Design review of the part built by this model. Coordinates are the model's own, in mm. Coordinates: 2 decimals unless noted, no trailing zeros. Loops run counter-clockwise (first coordinate to the right, second up) from the corner with the lowest first, then second, coordinate; pieces in that order, holes last. Notation, with made-up numbers: M -35.5,-24 L 10.5,-24 A36 cw 10.5,15 Z; hole C 59,86 d5. An arc over 180 degrees is marked long. Write item = value, one per line. Start each with the question number.
from build123d import *

# Parameters (mm, degrees)
F0_R     = 15.875
F0_R_2   = 11.25
F1_DEPTH = 38
F3_R     = 4
F4_DEPTH = 15.876


# Not quite as in the source:
# - a fillet or chamfer that OpenCascade refuses, or shapes differently, is made with other operations: its cross-section is extruded or revolved along the edge and cut away or added


with BuildPart() as f1:
    # F0 (on Top) → F1 (new body)
    with BuildSketch(Plane.XY):
        Circle(F0_R)
        Circle(F0_R_2, mode=Mode.SUBTRACT)
    extrude(amount=F1_DEPTH)

    # F2: fillet of radius 5 on 2 edges, made by hand

    # F2_s1 → F2_t2 (revolve, cut)
    with BuildSketch(Plane.XZ):
        with BuildLine():
            ThreePointArc((15.875, 33.0140823312), (14.5407195747, 36.4144499584), (11.25, 38))
            Line((11.25, 38), (15.875, 38))
            Line((15.875, 38), (15.875, 33.0140823312))
        make_face()
    revolve(axis=Axis((0, 0, 38), (0, 0, 1)), mode=Mode.SUBTRACT)

    # F2_s3 → F2_t4 (revolve, cut)
    with BuildSketch(Plane.XZ):
        with BuildLine():
            ThreePointArc((15.875, 4.9859176688), (14.5407195747, 1.5855500416), (11.25, 0))
            Line((11.25, 0), (15.875, 0))
            Line((15.875, 0), (15.875, 4.9859176688))
        make_face()
    revolve(axis=Axis((0, 0, 0), (0, 0, 1)), mode=Mode.SUBTRACT)

    # F3 (on Front) → F4 (cut, through all)
    with BuildSketch(Plane.XZ):
        with Locations((0, 12)):
            Circle(F3_R)
        with Locations((0, 26)):
            Circle(F3_R)
    extrude(amount=-F4_DEPTH, mode=Mode.SUBTRACT)


solid = f1.part
Q1. Add section B-B on x = 0. State the section outline as (y, z) points (3 decimals).
Q2. To check wall thickness, follow line 1 (Z direction, x = 0, y = 11.85); line 2 (Z direction, x = 0, y = 13); line 3 (X direction, y = 0.5, z = 11.5). State the ranges of each line that lie inside material, in increasing order. Write a range as from..to.
Q3. Add section C-C on z = 35. State the section outline as (x, y) points.
Q4. Clearance check with flat-ended pins moving along their axes: P1, Ø1.5, axis at x = -5, z = 26, coming from the +Y side; P2, Ø10, axis at y = -11.5, z = 23, coming from the -X side; P3, Ø5, axis at y = 8.5, z = 13, coming from the +X side. State where each tip first meets the part, or that it passes through.
Q5. Mouldability with a two-part tool opening along X and no side actions: class faces 1 (the face through (-0.521, 13.157, 15.966)), 2 (the face through (-3.441, -15.497, 18.804)), 3 (the face through (5.19, -9.98, 18.73)) as released by +X, released by -X, zero draft, split by the parting line, or undercut.
Q6. Add section D-D on z = 26. State the section outline as (x, y) points (3 decimals).
Q7. Add section A-A on y = 0. State the section outline as (x, z) points (3 decimals), plus the area to 3 significant figures.
Values follow:
q1.outline = M -15.875,4.986 A5 ccw -11.25,0 L -11.25,38 A5 ccw -15.875,33.014 Z; M 11.25,0 A5 ccw 15.875,4.986 L 15.875,8 L 11.25,8 Z; M 11.25,16 L 15.875,16 L 15.875,22 L 11.25,22 Z; M 11.25,30 L 15.875,30 L 15.875,33.014 A5 ccw 11.25,38 Z
q2.line_1 = 0.08..8, 16..22, 30..37.92
q2.line_2 = 0.46..8, 16..22, 30..37.54
q2.line_3 = -15.87..-11.24, 11.24..15.87
q3.outline = C 0,0 d30.93; hole C 0,0 d22.5
q4.P1 = 15.3
q4.P2 = -14.48
q4.P3 = 14.7
q5.face_1 = undercut
q5.face_2 = split by the parting line
q5.face_3 = undercut
q6.outline = M -4,10.515 L -4,15.363 A15.875 ccw long 4,15.363 L 4,10.515 A11.25 cw long Z
q7.outline = M -15.875,4.986 A5 ccw -11.25,0 L -11.25,38 A5 ccw -15.875,33.014 Z; M 11.25,0 A5 ccw 15.875,4.986 L 15.875,33.014 A5 ccw 11.25,38 Z
q7.area = 330 mm2
